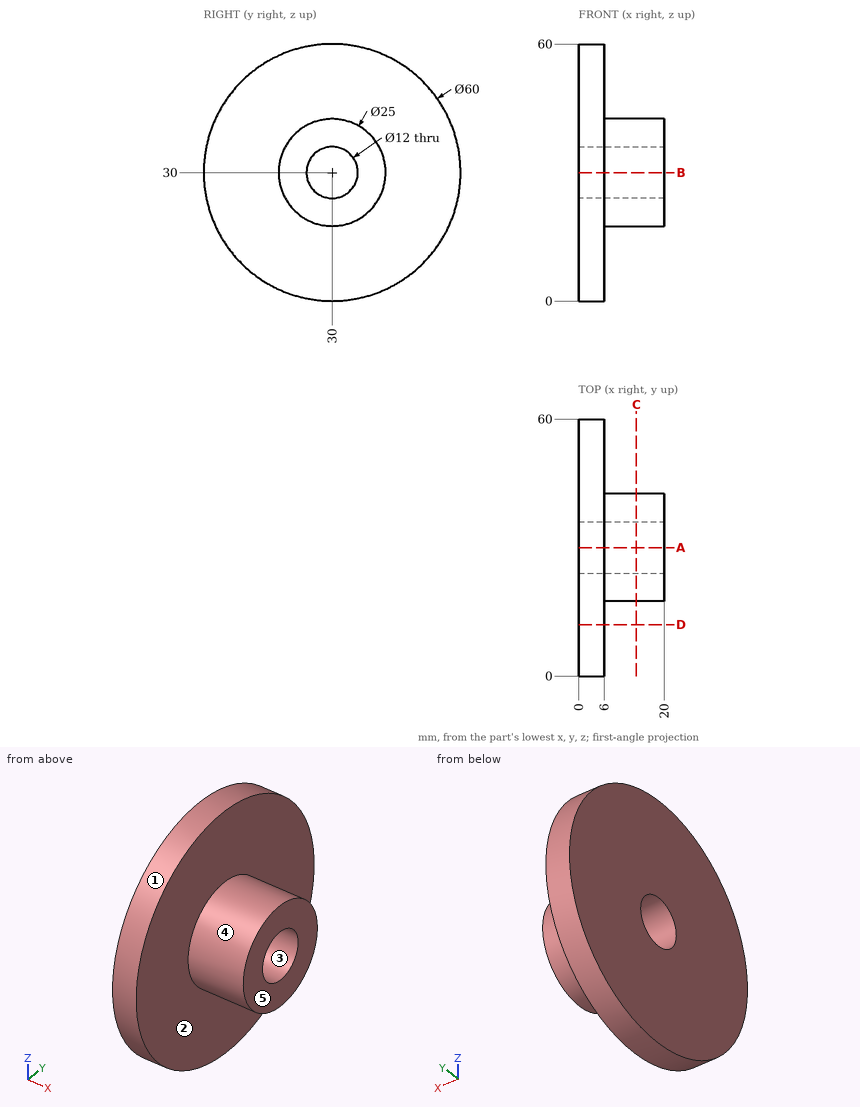
Geometry check sheet. Reference: drawing and pictorial views, mm from the part's lowest x, y, z. A direction names the side the tool comes from. Round coordinates to 2 decimals unless told otherwise and drop trailing zeros. Order: outer loops, then holes, each group sorted by start corner. A loop starts at its lowest first (then second) coordinate and runs counter-clockwise, first axis right, second up. Notation, with made-up numbers: M 81.5,-6 L 139.5,-6 A15 ccw 139.5,22 Z; hole C 4,29 d8. An arc over 180 degrees is marked long. Answer as CSV lines item,"result".
1) Gauge pin test, flat ends, axial feed: pin 1 Ø2 at (x, y) = (6.5, 17.5) entering from +Z; pin 2 Ø7 at (y, z) = (30, 30) entering from -X; pin 3 Ø1 at (x, y) = (12.5, 28) entering from -Z; pin 4 Ø2 at (y, z) = (18, 18) entering from +X. Record the tip position at first contact, or that the pin passes through.
Entries:
pin 1,"z = 57.65"
pin 2,"through"
pin 3,"z = 17.59"
pin 4,"x = 6"
2) Mould release check, pull along Z, two halves, no side actions. Record for the marked faces 1, 2 and 3: +Z half, -Z half, draft (parallel to the pull), parting line (faces both ways), or undercut.
Entries:
face 1,"parting line"
face 2,"draft"
face 3,"undercut"
3) Sectioned sample at D-D on y = 12. Record the cut outline in (x, z).
Entries:
outline,"M 0,6 L 6,6 L 6,54 L 0,54 Z"
4) Thickness scan on probe 1 along Y at (x, z) = (12, 30); probe 2 along X at (y, z) = (40, 43.5); probe 3 along Z at (x, y) = (8.25, 27). Record the ranges inside material, lowest first. Write a range as [from, to].
Entries:
probe 1,"[17.5, 24], [36, 42.5]"
probe 2,"[0, 6]"
probe 3,"[17.87, 24.8], [35.2, 42.13]"
5) Tool access check on the marked faces 4 and 5. Record the directions out of +Z, -Z, +X, -X, +Y, -Y that give a thin tool (end or side, any length) a straight path to the whole face; none if there is none.
Entries:
face 4,"+X"
face 5,"+Z, -Z, +X, +Y, -Y"
6) Sectioned sample at A-A on y = 30. Record the cut outline in (x, z).
Entries:
outline,"M 0,0 L 6,0 L 6,17.5 L 20,17.5 L 20,24 L 0,24 Z; M 0,36 L 20,36 L 20,42.5 L 6,42.5 L 6,60 L 0,60 Z"
7) Sectioned sample at C-C on x = 13.5. Record the cut outline in (y, z), and give its area (3 significant figures).
Entries:
outline,"C 30,30 d25; hole C 30,30 d12"
area,"378 mm2"
